Can you work these out from the model? Positions are in its coordinate system, mm. Face numbers are marked on the shaded views. A direction names the side the tool comes from. Coordinates: 2 decimals unless noted, no trailing zeros. Loops run counter-clockwise (first coordinate to the right, second up) from the corner with the lowest first, then second, coordinate; pieces in that order, holes last. Notation, with made-up numbers: (0, -31) - (5, -31) arc R31 cw to (5, -7) - close; hole circle Ø4 at (-40, -8). An arc over 180 degrees is marked (long way). Put each result on its own line as item: value. Start each with the question number.
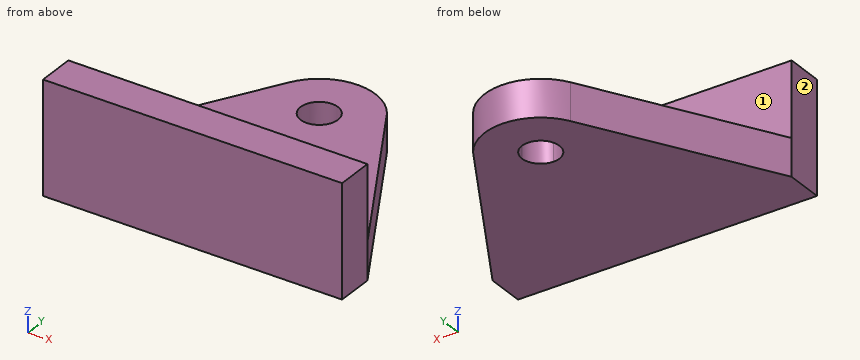
from build123d import *

# Parameters (mm, degrees)
EXTRUDE_1_DEPTH = 2
SKETCH_2_W      = 16
SKETCH_2_H      = 2
EXTRUDE_2_DEPTH = 6


with BuildPart() as part:
    # 草图1 → 凸台-拉伸1 (new body)
    with BuildSketch(Plane.XY):
        with BuildLine():
            Line((-8, -8), (0, -8))
            Line((0, -8), (8, -8))
            Line((8, -8), (2.719740406, 1.26610115))
            Line((2.719740406, 1.26610115), (2.475636513, 1.694468606))
            ThreePointArc((2.475636513, 1.694468606), (-0.124757283, 2.997404814), (-2.607883521, 1.482883521))
            Line((-2.607883521, 1.482883521), (-8, -8))
        make_face()
        with BuildLine():
            ThreePointArc((0, -1), (-0.707106781, 0.707106781), (1, 0))
            ThreePointArc((1, 0), (0.707106781, -0.707106781), (0, -1))
        make_face(mode=Mode.SUBTRACT)
    extrude(amount=EXTRUDE_1_DEPTH)

    # 草图2 → 凸台-拉伸2 (add)
    with BuildSketch(Plane(origin=(0, 0, 0), x_dir=(-1, 0, 0), z_dir=(0, 0, -1))):
        with Locations((0, -9)):
            Rectangle(SKETCH_2_W, SKETCH_2_H)
    extrude(amount=-EXTRUDE_2_DEPTH)


solid = part.part
Q1. Please list where these lines run through material, in increasing order: line 1 along Y through (x, z) = (0.75, 2.25); line 2 along Z through (x, y) = (2.25, -3.25); line 3 along X through (y, z) = (-2, 1.3). Write a range as [from, to].
Q2. On a 3-axis mill with a long thin cutter (end or side, diameter ignored), from which of +Z, -Z, +X, -X, +Y, -Y can I reach the whole of each face in a straight line? I mean the marked faces 1 and 2. Say none if no direction works.
Q3. Will these pins go through, and if not, where does the flat tip stop? pin 1 (3 mm diameter, centred on x = 5, y = 0, fed in from +Z); pin 2 (1 mm diameter, centred on x = 2, y = 1.5, fed in from -Z); pin 3 (3 mm diameter, centred on x = 2, z = 4, fed in from +Y).
Q4. I want a section at B-B on x = -4. List the corners of the cut face in (y, z) for me, and give its area (3 significant figures).
Q5. I want a section at C-C on y = -7.5. List the corners of the cut face in (x, z) for me.
Q6. I want a section at D-D on z = 2.3. List the corners of the cut face in (x, y) for me.
Q7. I want a section at A-A on z = 1. List the corners of the cut face in (x, y) for me, and give its area (3 significant figures).
Calculated:
1. line 1: [-10, -8]
1. line 2: [0, 2]
1. line 3: [-4.59, 4.58]
2. face 1: +Z, +X, -X, +Y
2. face 2: +Z, -Z, -X, +Y, -Y
3. pin 1: z = 2
3. pin 2: z = 0
3. pin 3: y = -8
4. outline: (-10, 0) - (-0.97, 0) - (-0.97, 2) - (-8, 2) - (-8, 6) - (-10, 6) - close
4. area: 26.1 mm2
5. outline: (-7.72, 0) - (7.72, 0) - (7.72, 2) - (-7.72, 2) - close
6. outline: (-8, -10) - (8, -10) - (8, -8) - (-8, -8) - close
7. outline: (-8, -10) - (8, -10) - (8, -8) - (2.48, 1.69) arc R3 ccw to (-2.61, 1.48) - (-8, -8) - close; hole circle Ø2 at (0, 0)
7. area: 135 mm2
